Model file for the job. Use its own axes, mm. A direction names the side the tool comes from. Give positions to 0.01 mm unless a question says otherwise; leave off trailing zeros. Loops run counter-clockwise (first coordinate to the right, second up) from the corner with the lowest first, then second, coordinate; pieces in that order, holes last. Notation, with made-up numbers: (59, -14.5) - (108, -14.5) arc R20 cw to (108, -6.5) - close; hole circle Ø11 at (76, 55). An arc over 180 degrees is marked (long way). Use a Markdown table: item, result.
from build123d import *

# Parameters (mm, degrees)
BOSS_EXTRUDE1_DEPTH      = 1.25
SKETCH2_W                = 1
SKETCH2_H                = 0.325
BOSS_EXTRUDE2_DEPTH      = 2
SKETCH3_W                = 1
SKETCH3_H                = 0.325
BOSS_EXTRUDE3_DEPTH      = 2
BOSS_EXTRUDE7_DEPTH      = 1
BOSS_EXTRUDE8_DEPTH      = 1
SKETCH9_W                = 7
SKETCH9_H                = 0.624150965
BOSS_EXTRUDE9_DEPTH      = 12
BOSS_EXTRUDE9_DEPTH_BACK = 13.25


with BuildPart() as part:
    # Sketch1 → Boss-Extrude1 (new body)
    with BuildSketch(Plane.XY):
        Polygon((1, 0), (9, 0), (9, -0.325), (10, -0.325), (10, -1), (17, -1), (17, 1), (10, 1), (0, 1), (-7, 1), (-7, -1), (0, -1), (0, -0.325), (1, -0.325), align=None)
    extrude(amount=BOSS_EXTRUDE1_DEPTH)

    # Sketch2 → Boss-Extrude2 (add)
    with BuildSketch(Plane.XY.offset(1.25)):
        with Locations((0.5, -0.1625)):
            Rectangle(SKETCH2_W, SKETCH2_H)
        with Locations((9.5, -0.1625)):
            Rectangle(SKETCH2_W, SKETCH2_H)
    extrude(amount=BOSS_EXTRUDE2_DEPTH)

    # Sketch3 → Boss-Extrude3 (add)
    with BuildSketch(Plane(origin=(0, 0, 0), x_dir=(-1, 0, 0), z_dir=(0, 0, -1))):
        with Locations((-9.5, -0.1625)):
            Rectangle(SKETCH3_W, SKETCH3_H)
        with Locations((-0.5, -0.1625)):
            Rectangle(SKETCH3_W, SKETCH3_H)
    extrude(amount=BOSS_EXTRUDE3_DEPTH)

    # Sketch7 → Boss-Extrude7 (add)
    with BuildSketch(Plane(origin=(10, 0, 0), x_dir=(0, 0, -1), z_dir=(1, 0, 0))):
        Polygon((-3.25, 0), (-1.25, 1), (-1.25, 0), (-1.25, -0.325), (-3.25, -0.325), align=None)
        Polygon((2, 0), (0, 1), (0, 0), align=None)
    extrude(amount=-BOSS_EXTRUDE7_DEPTH)

    # Sketch8 → Boss-Extrude8 (add)
    with BuildSketch(Plane.ZY):
        Polygon((-2, 0), (0, 1), (0, 0), align=None)
        Polygon((1.25, 1), (1.25, 0), (3.25, 0), align=None)
    extrude(amount=-BOSS_EXTRUDE8_DEPTH)

    # Sketch9 → Boss-Extrude9 (add, two sides)
    with BuildSketch(Plane.XY.offset(1.25)) as boss_extrude9_sk:
        with Locations((-3.5, -0.687924517)):
            Rectangle(SKETCH9_W, SKETCH9_H)
        with Locations((13.5, -0.687924517)):
            Rectangle(SKETCH9_W, SKETCH9_H)
    extrude(amount=BOSS_EXTRUDE9_DEPTH)
    extrude(boss_extrude9_sk.sketch, amount=-BOSS_EXTRUDE9_DEPTH_BACK)


solid = part.part
(1) Slice it at D-D, the plane x = -2.25. Write the cut outline in (y, z).
Computed:
| item | result |
|---|---|
| outline | (-1, -12) - (-0.38, -12) - (-0.38, 0) - (1, 0) - (1, 1.25) - (-0.38, 1.25) - (-0.38, 13.25) - (-1, 13.25) - close |
(2) Slice it at A-A, the plane z = -4.25. Write the cut outline in (x, y), plus the area to 3 significant figures.
Computed:
| item | result |
|---|---|
| outline | (-7, -1) - (0, -1) - (0, -0.38) - (-7, -0.38) - close; (10, -1) - (17, -1) - (17, -0.38) - (10, -0.38) - close |
| area | 8.74 mm² |
(3) Drill centre lines: probe 1 along X at (y, z) = (-0.8, 1); probe 2 along X at (y, z) = (0.5, 1.75); probe 3 along Y at (x, z) = (-5.25, -0.25). Where is each one in solid material? Low to high. Write a range as [from, to].
Computed:
| item | result |
|---|---|
| probe 1 | [-7, 0], [10, 17] |
| probe 2 | [0, 1], [9, 10] |
| probe 3 | [-1, -0.38] |
(4) Mould opens along X. For faces 1 (the flat face through (10, 0, -1)), 2 (the flat face through (0, 0, 2)), 3 (the flat face through (-4, -0.376, -6)), 4 (the flat face through (0.5, -0.325, 0.7)) say: pulls with the +X half, pulls with the -X half, needs draft (parallel to the pull), parting line crosses it, or undercut.
Computed:
| item | result |
|---|---|
| face 1 | pulls with the +X half |
| face 2 | pulls with the -X half |
| face 3 | needs draft |
| face 4 | undercut |
(5) Slice it at C-C, the plane z = -1.25. Write the cut outline in (x, y) (3 decimals), plus the area to 3 significant figures.
Computed:
| item | result |
|---|---|
| outline | (-7, -1) - (0, -1) - (0, -0.376) - (-7, -0.376) - close; (0, -0.325) - (1, -0.325) - (1, 0.375) - (0, 0.375) - close; (9, -0.325) - (10, -0.325) - (10, 0.375) - (9, 0.375) - close; (10, -1) - (17, -1) - (17, -0.376) - (10, -0.376) - close |
| area | 10.1 mm² |
(6) Pin check, flat tips, straight feed: P1, Ø5.5, axis at x = 12.5, z = 6, coming from the +Y side; P2, Ø1.1, axis at x = 6, y = 0.5, coming from the +Z side. Stop position of each tip, or through.
Computed:
| item | result |
|---|---|
| P1 | y = -0.38 |
| P2 | z = 1.25 |
(7) Slice it at B-B, the plane y = -0.7. Write the cut outline in (x, z).
Computed:
| item | result |
|---|---|
| outline | (-7, -12) - (0, -12) - (0, 13.25) - (-7, 13.25) - close; (10, -12) - (17, -12) - (17, 13.25) - (10, 13.25) - close |
(8) 3-axis set-ups, long thin cutter, end or side, ignore diameter. For faces 5 (the flat face through (13, 0, 0)), 6 (the flat face through (13, -0.376, -6)), 7 (the flat face through (10, 0, 2)), 8 (the flat face through (0, 0, -1)), 9 (the flat face through (13, -0.376, 7)): which of +Z, -Z, +X, -X, +Y, -Y reach the whole face in a straight line?
Computed:
| item | result |
|---|---|
| face 5 | -Z, +X, +Y |
| face 6 | -Z, +X, -X, +Y |
| face 7 | +Z, +X, +Y |
| face 8 | -Z, -X, +Y |
| face 9 | +Z, +X, -X, +Y |
